Geometry check sheet. Reference: the model listing, model coordinates, mm. Face numbers are marked on the shaded views. A direction names the side the tool comes from. Round coordinates to 2 decimals unless told otherwise and drop trailing zeros. Write each loop counter-clockwise with the first axis right and the second up, starting at its lowest first coordinate (ties: lowest second). Pieces come first, ordered by that corner, then holes. Notation, with made-up numbers: (27, -10.5) - (47, -10.5) arc R9 cw to (47, -4.5) - close; hole circle Ø11 at (22.25, 67). An arc over 180 degrees is marked (long way). Return JSON: item names as keys, results as strings.
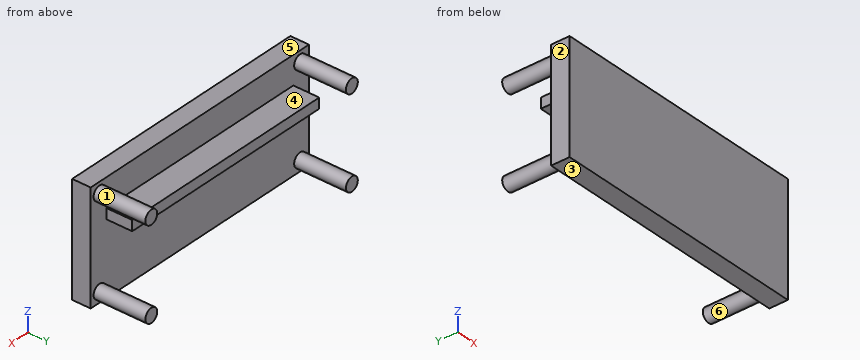
```python
from build123d import *

# Parameters (mm, degrees)
SKETCH1_W           = 70
SKETCH1_H           = 30
BOSS_EXTRUDE1_DEPTH = 15
SKETCH3_W           = 60
SKETCH3_H           = 2.8
BOSS_EXTRUDE3_DEPTH = 7
SKETCH4_W           = 70
SKETCH4_H           = 30
CUT_EXTRUDE1_DEPTH  = 10
SKETCH5_R           = 1.9
BOSS_EXTRUDE4_DEPTH = 14


with BuildPart() as part:
    # Sketch1 → Boss-Extrude1 (new body)
    with BuildSketch(Plane(origin=(0, 0, 0), x_dir=(1, 0, 0), z_dir=(0, 1, 0))):
        with Locations((35, 15)):
            Rectangle(SKETCH1_W, SKETCH1_H)
    extrude(amount=BOSS_EXTRUDE1_DEPTH)

    # Sketch3 → Boss-Extrude3 (add)
    with BuildSketch(Plane(origin=(0, 15, 0), x_dir=(1, 0, 0), z_dir=(0, 1, 0))):
        with Locations((35, 9)):
            Rectangle(SKETCH3_W, SKETCH3_H)
    extrude(amount=BOSS_EXTRUDE3_DEPTH)

    # Sketch4 → Cut-Extrude1 (cut)
    with BuildSketch(Plane(origin=(0, 0, 0), x_dir=(-1, 0, 0), z_dir=(0, -1, 0))):
        with Locations((-35, 15)):
            Rectangle(SKETCH4_W, SKETCH4_H)
    extrude(amount=-CUT_EXTRUDE1_DEPTH, mode=Mode.SUBTRACT)

    # Sketch5 → Boss-Extrude4 (add)
    with BuildSketch(Plane(origin=(0, 15, 0), x_dir=(1, 0, 0), z_dir=(0, 1, 0))):
        with Locations(Location((2.828427125, 2.828427125, 0), (0, 0, 90))):
            Circle(SKETCH5_R)
        with Locations(Location((2.828427125, 27.171572875, 0), (0, 0, 90))):
            Circle(SKETCH5_R)
        with Locations(Location((67.171572875, 27.171572875, 0), (0, 0, 90))):
            Circle(SKETCH5_R)
        with Locations(Location((67.171572875, 2.828427125, 0), (0, 0, 90))):
            Circle(SKETCH5_R)
    extrude(amount=BOSS_EXTRUDE4_DEPTH)


solid = part.part
```
(1) Material ranges on line 1 along Z through (x, y) = (3, 17.25); line 2 along Y through (x, z) = (23.5, -27.75); line 3 along Y through (x, z) = (49, -9.25), recorded low to high. Write a range as [from, to].
Response values:
{"line 1": "z = [-29.06, -25.28], [-4.72, -0.94]", "line 2": "y = [10, 15]", "line 3": "y = [10, 22]"}
(2) Section check D-D, the plane y = 25.5. Enter the section's corners in (x, z), plus the area to 3 significant figures.
Response values:
{"outline": "circle Ø3.8 at (2.83, -27.17); circle Ø3.8 at (2.83, -2.83); circle Ø3.8 at (67.17, -27.17); circle Ø3.8 at (67.17, -2.83)", "area": "45.4 mm^2"}
(3) Release check for a two-part mould opening along X. For the marked faces 1, 2 and 3 record: pulls with the +X half, pulls with the -X half, needs draft (parallel to the pull), parting line crosses it, or undercut.
Response values:
{"face 1": "undercut", "face 2": "pulls with the -X half", "face 3": "needs draft"}
(4) Section check B-B, the plane x = 4. Enter the section's corners in (y, z).
Response values:
{"outline": "(10, -30) - (15, -30) - (15, -28.67) - (29, -28.67) - (29, -25.68) - (15, -25.68) - (15, -4.32) - (29, -4.32) - (29, -1.33) - (15, -1.33) - (15, 0) - (10, 0) - close"}
(5) Section check A-A, the plane y = 16. Enter the section's corners in (x, z).
Response values:
{"outline": "circle Ø3.8 at (2.83, -27.17); circle Ø3.8 at (2.83, -2.83); (5, -10.4) - (65, -10.4) - (65, -7.6) - (5, -7.6) - close; circle Ø3.8 at (67.17, -27.17); circle Ø3.8 at (67.17, -2.83)"}
(6) Gauge pin test, flat ends, axial feed: pin 1 (9 mm diameter, centred on x = 49.5, z = -21, fed in from +Y); pin 2 (0.8 mm diameter, centred on x = 33.5, z = -9.5, fed in from +Y); pin 3 (2 mm diameter, centred on y = 17, z = -9, fed in from -X); pin 4 (2 mm diameter, centred on y = 25.5, z = -24, fed in from -X) (3 decimals). Record the tip position at first contact, or that the pin passes through.
Response values:
{"pin 1": "stops at y = 15", "pin 2": "stops at y = 22", "pin 3": "stops at x = 5", "pin 4": "passes through"}
(7) Section check C-C, the plane z = -3.5. Enter the section's corners in (x, y), plus the area to 3 significant figures.
Response values:
{"outline": "(0, 10) - (70, 10) - (70, 15) - (68.95, 15) - (68.95, 29) - (65.39, 29) - (65.39, 15) - (4.61, 15) - (4.61, 29) - (1.05, 29) - (1.05, 15) - (0, 15) - close", "area": "450 mm^2"}
(8) Access from +Z, -Z, +X, -X, +Y, -Y to the whole of each face (thin tool, end or side, straight path). Record for the marked faces 4, 5 and 6.
Response values:
{"face 4": "+Z, +X, -X, +Y", "face 5": "+Z, +X, -X, +Y, -Y", "face 6": "+Y"}
